```python
from build123d import *

# Parameters (mm, degrees)
F0_R     = 30
F1_DEPTH = 50
F2_T     = -2.75
F3_W     = 10
F3_H     = 10
F4_DEPTH = 30
F5_W     = 12
F5_H     = 10
F6_DEPTH = 50


with BuildPart() as f1:
    # F0 (on Top) → F1 (new body)
    with BuildSketch(Plane.XY):
        Circle(F0_R)
    extrude(amount=F1_DEPTH)

    # F2
    f2_openings = [f1.faces().sort_by_distance(p)[0] for p in [
        (0, 0, 50),
    ]]
    offset(amount=F2_T, openings=f2_openings)

    # F3 (on Front) → F4 (cut, symmetric)
    with BuildSketch(Plane.XZ):
        with Locations((-22.25, 42.25)):
            Rectangle(F3_W, F3_H)
        with Locations((-22.25, 27.75)):
            Rectangle(F3_W, F3_H)
        with Locations((-22.25, 13.25)):
            Rectangle(F3_W, F3_H)
        with Locations((-7.75, 42.25)):
            Rectangle(F3_W, F3_H)
        with Locations((-7.75, 27.75)):
            Rectangle(F3_W, F3_H)
        with Locations((-7.75, 13.25)):
            Rectangle(F3_W, F3_H)
        with Locations((6.75, 42.25)):
            Rectangle(F3_W, F3_H)
        with Locations((6.75, 27.75)):
            Rectangle(F3_W, F3_H)
        with Locations((6.75, 13.25)):
            Rectangle(F3_W, F3_H)
        with Locations((21.25, 42.25)):
            Rectangle(F3_W, F3_H)
        with Locations((21.25, 27.75)):
            Rectangle(F3_W, F3_H)
        with Locations((21.25, 13.25)):
            Rectangle(F3_W, F3_H)
    extrude(amount=F4_DEPTH, both=True, mode=Mode.SUBTRACT)

    # F5 (on Right) → F6 (cut, symmetric)
    with BuildSketch(Plane.YZ):
        with Locations((0, 13.25)):
            Rectangle(F5_W, F5_H)
        with Locations((0, 27.75)):
            Rectangle(F5_W, F5_H)
        with Locations((0, 42.25)):
            Rectangle(F5_W, F5_H)
    extrude(amount=F6_DEPTH, both=True, mode=Mode.SUBTRACT)


solid = f1.part
```
CAD build for the part. Positions are in the model's coordinates, mm. A direction names the side the tool comes from. Give positions to 0.01 mm unless a question says otherwise; leave off trailing zeros. Order: outer loops, then holes, each group sorted by start corner. A loop starts at its lowest first (then second) coordinate and runs counter-clockwise, first axis right, second up.
(1) Saw through at D-D, the plane x = -15. Give the cut face in (y, z), then the cut area to 3 significant figures.
(2) Drill centre lines: L1, parallel to Z at x = -27, y = 12; L2, parallel to Y at x = 0, z = 38; L3, parallel to Z at x = 21.5, y = 6. Where is each one in solid material? Low to high.
(3) Saw through at A-A, the plane y = 0. State how many separate pieces and enclosed holes the cut face has, then the cut area to 3 significant figures.
(4) Tool access for faces 4 (the flat face through (-27.4, -1.7, 47.25)), 5 (the flat face through (-17.25, 23, 28)), 6 (the flat face through (-12.75, -26, 42)), 7 (the flat face through (28, 0, 8.25)): list every direction of +Z, -Z, +X, -X, +Y, -Y with a clear straight run to the whole face (end or side of a thin tool).
(5) Mould opens along Z. For faces 1 (the flat face through (28, 6, 42)), 2 (the flat face through (-8, 28, 47.25)), 3 (the flat face through (0, 0, 0)) say: released by +Z, released by -Z, zero draft, split by the parting line, or undercut.
(6) Saw through at B-B, the plane x = 0. Give the cut face in (y, z).
(7) Flat gauge pins, fed straight in: pin 1 (6 mm diameter, centred on x = 6, y = 27, fed in from -Z); pin 2 (3.5 mm diameter, centred on y = 26.5, z = 43.5, fed in from -X); pin 3 (1 mm diameter, centred on x = 24, z = 28.5, fed in from +Y); pin 4 (1.5 mm diameter, centred on y = -26.5, z = 11, fed in from -X). Where does each tip first touch, or does it go through?
Results found:
1. outline: (-25.98, 0) - (25.98, 0) - (25.98, 50) - (22.75, 50) - (22.75, 2.75) - (-22.75, 2.75) - (-22.75, 50) - (-25.98, 50) - close
1. area: 448 mm2
2. L1: z = 0 to 8.25, 18.25 to 22.75, 32.75 to 37.25, 47.25 to 50
2. L2: y = -30 to -27.25, 27.25 to 30
2. L3: z = 0 to 2.75
3. separate pieces: 7
3. enclosed holes: 0
3. area: 260 mm2
4. face 4: none
4. face 5: -X, +Y, -Y
4. face 6: +Y, -Y
4. face 7: +X, -X
5. face 1: undercut
5. face 2: undercut
5. face 3: released by -Z
6. outline: (-30, 0) - (30, 0) - (30, 50) - (27.25, 50) - (27.25, 2.75) - (-27.25, 2.75) - (-27.25, 50) - (-30, 50) - close
7. pin 1: stops at z = 0
7. pin 2: stops at x = -16.95
7. pin 3: passes through
7. pin 4: stops at x = -15.39
